Check sheet for the modelled part. Datum: model origin and axes. Units: mm. Round coordinates to 2 decimals unless told otherwise and drop trailing zeros. Write each loop counter-clockwise with the first axis right and the second up, starting at its lowest first coordinate (ties: lowest second). Pieces come first, ordered by that corner, then holes. Notation, with made-up numbers: (27.25, 49.5) -> (64.25, 49.5) arc R21 cw to (64.25, 62.5) -> close; hole circle Ø5 at (-34.5, 75.5). An arc over 180 degrees is marked (long way). Answer as a JSON object with one key per item and string values. Group by question number.
Autodesk Inventor part; units mm, degrees
ref_plane "YZ Plane" through (0, 0, 0) normal (1, 0, 0) x (0, 1, 0)
ref_plane "XZ Plane" through (0, 0, 0) normal (0, 1, 0) x (-1, 0, 0)
ref_plane "XY Plane" through (0, 0, 0) normal (0, 0, 1) x (1, 0, 0)
sketch "Sketch1" plane through (0, 0, 0) normal (0, 0, 1) x (1, 0, 0)
  line L0 (0.0202, 5.1733) -> (0.0202, -4.6267)
  line L1 (0.6202, 5.1733) -> (0.6202, 4.1733)
  line L2 (1.2202, 3.2495) -> (1.2202, -2.703)
  line L3 (0.6202, 4.1733) -> (1.2202, 4.1733)
  line L4 (0.0202, 5.1733) -> (0.6202, 5.1733)
  line L5 (1.2202, 4.1733) -> (2.2202, 4.7506)
  line L6 (1.2202, 3.2495) -> (2.2202, 3.8268)
  line L7 (3.2202, 4.1733) -> (2.2202, 4.7506)
  line L8 (3.2202, 3.2495) -> (2.2202, 3.8268)
  line L9 (3.2202, 3.2495) -> (3.2202, 4.1733)
  line L10 (0.6202, -4.6267) -> (0.6202, -3.6267)
  line L11 (0.6202, -3.6267) -> (1.2202, -3.6267)
  line L12 (0.0202, -4.6267) -> (0.6202, -4.6267)
  line L13 (1.2202, -3.6267) -> (2.2202, -4.2041)
  line L14 (1.2202, -2.703) -> (2.2202, -3.2803)
  line L15 (3.2202, -3.6267) -> (2.2202, -4.2041)
  line L16 (3.2202, -2.703) -> (2.2202, -3.2803)
  line L17 (3.2202, -2.703) -> (3.2202, -3.6267)
  point P0 (0, 0)
  dimension "d0" = 120
  dimension "d1" = 120
  dimension "d2" = 90
  dimension "d3" = 60
  dimension "d4" = 2
  dimension "d5" = 2.6
  dimension "d6" = 3.2
  dimension "d7" = 0.8
  dimension "d8" = 6.955
  dimension "d9" = 7.755
  dimension "d10" = 0.8
  dimension "d11" = 6.955
  dimension "d12" = 6.155
  dimension "d13" = 7.8
  dimension "d14" = 1
  dimension "d15" = 8.8
  dimension "d16" = 3.2202
  dimension "d17" = 3.2202
  dimension "d18" = 5.2242
  dimension "d19" = 3.951
  dimension "d20" = 4.1733
  dimension "d21" = 0.6202
extrude "Extrusion1" add sketch "Sketch1" along normal mid plane 250
properties part number "T Slot Cover 250mm" material "PC/ABS Plastic"
(1) Release check for a two-part mould opening along Y. For faces 1 (the flat face through (0.02, 0, -2)), 2 (the flat face through (1.22, 0, -2)) record: pulls with the +Y half, pulls with the -Y half, needs draft (parallel to the pull), parting line crosses it, or undercut.
(2) Section check A-A on z = -60.5. Record the cut outline in (x, y).
(3) Go/stop test with flat-tipped pins: pin 1 Ø1.5 at (x, z) = (1.5, -94.5) entering from +Y; pin 2 Ø1 at (x, y) = (2.5, 2.5) entering from -Z; pin 3 Ø5 at (y, z) = (0, -58.5) entering from +X; pin 4 Ø0.5 at (y, z) = (-4, 61.5) entering from +X. Record where each tip stops, or that it passes through.
(4) Scan lines: line 1 along X through (y, z) = (2, -104.5); line 2 along Y through (x, z) = (1.7, 49); line 3 along X through (y, z) = (4.25, 21.5). Record each from-to range of solid material in increasing order.
Data:
{
 "1": {"face 1": "needs draft", "face 2": "undercut"},
 "2": {"outline": "(0.02, -4.63) -> (0.62, -4.63) -> (0.62, -3.63) -> (1.22, -3.63) -> (2.22, -4.2) -> (3.22, -3.63) -> (3.22, -2.7) -> (2.22, -3.28) -> (1.22, -2.7) -> (1.22, 3.25) -> (2.22, 3.83) -> (3.22, 3.25) -> (3.22, 4.17) -> (2.22, 4.75) -> (1.22, 4.17) -> (0.62, 4.17) -> (0.62, 5.17) -> (0.02, 5.17) -> close"},
 "3": {"pin 1": "stops at y = 4.75", "pin 2": "passes through", "pin 3": "stops at x = 1.22", "pin 4": "stops at x = 3.01"},
 "4": {"line 1": "x = 0.02 to 1.22", "line 2": "y = -3.9 to -2.98, 3.53 to 4.45", "line 3": "x = 0.02 to 0.62, 1.35 to 3.09"}
}
